Here's how the part is built. I have some questions about the finished solid (model axes, mm). A direction names the side the tool comes from. Give positions to 0.01 mm unless a question says otherwise; leave off trailing zeros. Order: outer loops, then holes, each group sorted by start corner. A loop starts at its lowest first (then second) coordinate and runs counter-clockwise, first axis right, second up. Notation, with made-up numbers: (-24.5, 12.5) -> (13.5, 12.5) arc R32 ccw to (13.5, 47.5) -> close; hole circle Ø1 at (0, 24). An arc over 180 degrees is marked (long way). Write each question's results on one line, items separated by ' | '. Start each with the question number.
Q1. Imagine slicing it at A-A, the plane y = 10.75. Please give me the cut outline in (x, z), then the cut area to 3 significant figures.
Q2. Imagine slicing it at B-B, the plane x = 44. Please give me the cut outline in (y, z).
Q3. Thinking about a two-plate mould opening in Y: for faces 1 (the face through (-2, 26.2, 0.5)), 2 (the face through (58, 0, 12)), 3 (the face through (56.3, 0.06, 6.42)), 4 (the face through (-2.1, -2, 0.5)), which applies, pulls with the +Y half, pulls with the -Y half, needs draft (parallel to the pull), parting line crosses it, or undercut?
Q4. I need wall thicknesses on line 1 along X through (y, z) = (4, 0.75); line 2 along X through (y, z) = (0, 6.25); line 3 along Z through (x, y) = (4.5, 25). Which ranges of each line are inside material? Lowest first, please. Write a range as [from, to].
Q5. For faces 5 (the face through (-1.4, 0.06, 6.42)), 6 (the face through (21.3, 12.3, 0)), which set-ups out of +Z, -Z, +X, -X, +Y, -Y let a thin tool reach every point of the face, with its end or its side?
Q6. Imagine slicing it at D-D, the plane y = 5.25. Please give me the cut outline in (x, z), then the cut area to 3 significant figures.
Q7. I'm going to push flat-ended pins straight in: pin 1 (1 mm diameter, centred on y = 22.5, z = 10, fed in from -X); pin 2 (0.8 mm diameter, centred on x = 58, z = 0.5, fed in from -Y); pin 3 (6 mm diameter, centred on y = 17, z = 10.5, fed in from +X); pin 4 (6 mm diameter, centred on x = 22, y = 1, fed in from +Z). Where does each tip first touch, or does it pass through?
Q8. Imagine slicing it at C-C, the plane z = 8. Please give me the cut outline in (x, y), then the cut area to 3 significant figures.
```python
from build123d import *

# Parameters (mm, degrees)
EXTRUDE_1_DEPTH     = 1
SKETCH_2_R          = 1.4
EXTRUDE_2_DEPTH     = 12
SKETCH_10_W         = 17.6
SKETCH_10_H         = 16
SKETCH_10_W_2       = 6.2
SKETCH_10_H_2       = 11
SKETCH_10_W_3       = 26.5
SKETCH_10_H_3       = 19.9
CUT_EXTRUDE_1_DEPTH = 2


with BuildPart() as part:
    # 草图1 → 凸台-拉伸1 (new body)
    with BuildSketch(Plane.XY):
        with BuildLine():
            Line((0, -2.9), (57.7, -2.9))
            ThreePointArc((57.7, -2.9), (59.750609665, -2.050609665), (60.6, 0))
            Line((60.6, 0), (60.6, 24.1))
            ThreePointArc((60.6, 24.1), (59.750609665, 26.150609665), (57.7, 27))
            Line((57.7, 27), (0, 27))
            ThreePointArc((0, 27), (-2.050609665, 26.150609665), (-2.9, 24.1))
            Line((-2.9, 24.1), (-2.9, 0))
            ThreePointArc((-2.9, 0), (-2.050609665, -2.050609665), (0, -2.9))
        make_face()
    extrude(amount=EXTRUDE_1_DEPTH)

    # 草图2 → 凸台-拉伸2 (add)
    with BuildSketch(Plane.XY):
        with Locations((0, 24.1)):
            Circle(SKETCH_2_R)
        Circle(SKETCH_2_R)
        with Locations((57.7, 0)):
            Circle(SKETCH_2_R)
        with Locations((57.7, 24.1)):
            Circle(SKETCH_2_R)
    extrude(amount=EXTRUDE_2_DEPTH)

    # 草图10 → 切除-拉伸1 (cut, through all)
    with BuildSketch(Plane.XY.offset(1)):
        with Locations((12.15, 12.05)):
            Rectangle(SKETCH_10_W, SKETCH_10_H)
        with Locations((57.5, 11.6)):
            Rectangle(SKETCH_10_W_2, SKETCH_10_H_2)
        with Locations((37.85, 10.05)):
            Rectangle(SKETCH_10_W_3, SKETCH_10_H_3)
    extrude(amount=-CUT_EXTRUDE_1_DEPTH, mode=Mode.SUBTRACT)


solid = part.part
```
Geometry check:
1) outline: (-2.9, 0) -> (3.35, 0) -> (3.35, 1) -> (-2.9, 1) -> close; (20.95, 0) -> (24.6, 0) -> (24.6, 1) -> (20.95, 1) -> close; (51.1, 0) -> (54.4, 0) -> (54.4, 1) -> (51.1, 1) -> close | area: 13.2 mm²
2) outline: (-2.9, 0) -> (0.1, 0) -> (0.1, 1) -> (-2.9, 1) -> close; (20, 0) -> (27, 0) -> (27, 1) -> (20, 1) -> close
3) face 1: pulls with the +Y half | face 2: needs draft | face 3: undercut | face 4: pulls with the -Y half
4) line 1: [-2.9, 24.6], [51.1, 60.6] | line 2: [-1.4, 1.4], [56.3, 59.1] | line 3: [0, 1]
5) face 5: +Z | face 6: -Z, +X, -X, +Y, -Y
6) outline: (-2.9, 0) -> (3.35, 0) -> (3.35, 1) -> (-2.9, 1) -> close; (20.95, 0) -> (24.6, 0) -> (24.6, 1) -> (20.95, 1) -> close; (51.1, 0) -> (60.6, 0) -> (60.6, 1) -> (51.1, 1) -> close | area: 19.4 mm²
7) pin 1: x = -0.87 | pin 2: y = -2.9 | pin 3: through | pin 4: z = 1
8) outline: circle Ø2.8 at (0, 0); circle Ø2.8 at (0, 24.1); circle Ø2.8 at (57.7, 0); circle Ø2.8 at (57.7, 24.1) | area: 24.6 mm²
